from build123d import *

# Parameters (mm, degrees)
BOSS_EXTRUDE1_DEPTH = 5
SKETCH2_R           = 1.95
SKETCH2_W           = 40
SKETCH2_H           = 20
CUT_EXTRUDE1_DEPTH  = 6
SKETCH4_W           = 22
SKETCH4_H           = 49.22
CUT_EXTRUDE2_DEPTH  = 10
FILLET1_R           = 2
FILLET2_R           = 2
FILLET3_R           = 2
FILLET4_R           = 2
SKETCH5_R           = 1.95
SKETCH5_R_2         = 2
CUT_EXTRUDE3_DEPTH  = 6


with BuildPart() as part:
    # Sketch1 → Boss-Extrude1 (new body)
    with BuildSketch(Plane(origin=(0, 0, 0), x_dir=(1, 0, 0), z_dir=(0, 1, 0))):
        with BuildLine():
            Line((2, 0), (98, 0))
            ThreePointArc((98, 0), (99.414213562, -0.585786438), (100, -2))
            Line((100, -2), (100, -47.22))
            ThreePointArc((100, -47.22), (99.414213562, -48.634213562), (98, -49.22))
            Line((98, -49.22), (2, -49.22))
            ThreePointArc((2, -49.22), (0.585786438, -48.634213562), (0, -47.22))
            Line((0, -47.22), (0, -2))
            ThreePointArc((0, -2), (0.585786438, -0.585786438), (2, 0))
        make_face()
    extrude(amount=BOSS_EXTRUDE1_DEPTH)

    # Sketch2 → Cut-Extrude1 (cut, through all)
    with BuildSketch(Plane(origin=(0, 5, 0), x_dir=(1, 0, 0), z_dir=(0, 1, 0))):
        with Locations((90, -4.00475022)):
            Circle(SKETCH2_R)
        with Locations((82, -4.00475022)):
            Circle(SKETCH2_R)
        with Locations((18, -4.00475022)):
            Circle(SKETCH2_R)
        with Locations((26, -4.00475022)):
            Circle(SKETCH2_R)
        with Locations((34, -4.00475022)):
            Circle(SKETCH2_R)
        with Locations((42, -4.00475022)):
            Circle(SKETCH2_R)
        with Locations((50, -4.00475022)):
            Circle(SKETCH2_R)
        with Locations((58, -4.00475022)):
            Circle(SKETCH2_R)
        with Locations((66, -4.00475022)):
            Circle(SKETCH2_R)
        with Locations((74, -4.00475022)):
            Circle(SKETCH2_R)
        with Locations((90, -45.22)):
            Circle(SKETCH2_R)
        with Locations((82, -45.22)):
            Circle(SKETCH2_R)
        with Locations((18, -45.22)):
            Circle(SKETCH2_R)
        with Locations((26, -45.22)):
            Circle(SKETCH2_R)
        with Locations((34, -45.22)):
            Circle(SKETCH2_R)
        with Locations((42, -45.22)):
            Circle(SKETCH2_R)
        with Locations((50, -45.22)):
            Circle(SKETCH2_R)
        with Locations((58, -45.22)):
            Circle(SKETCH2_R)
        with Locations((66, -45.22)):
            Circle(SKETCH2_R)
        with Locations((74, -45.22)):
            Circle(SKETCH2_R)
        with Locations((50, -24.61)):
            Rectangle(SKETCH2_W, SKETCH2_H)
    extrude(amount=-CUT_EXTRUDE1_DEPTH, mode=Mode.SUBTRACT)

    # Sketch4 → Cut-Extrude2 (cut)
    with BuildSketch(Plane(origin=(0, 5, 0), x_dir=(1, 0, 0), z_dir=(0, 1, 0))):
        with Locations((89, -24.61)):
            Rectangle(SKETCH4_W, SKETCH4_H)
        with Locations((11, -24.61)):
            Rectangle(SKETCH4_W, SKETCH4_H)
    extrude(amount=-CUT_EXTRUDE2_DEPTH, mode=Mode.SUBTRACT)

    # Fillet1
    fillet1_edges = [part.edges().sort_by_distance(p)[0] for p in [
        (22, 2.5, 0),
    ]]
    fillet(fillet1_edges, radius=FILLET1_R)

    # Fillet2
    fillet2_edges = [part.edges().sort_by_distance(p)[0] for p in [
        (22, 2.5, 49.22),
    ]]
    fillet(fillet2_edges, radius=FILLET2_R)

    # Fillet3
    fillet3_edges = [part.edges().sort_by_distance(p)[0] for p in [
        (78, 2.5, 49.22),
    ]]
    fillet(fillet3_edges, radius=FILLET3_R)

    # Fillet4
    fillet4_edges = [part.edges().sort_by_distance(p)[0] for p in [
        (78, 2.5, 0),
    ]]
    fillet(fillet4_edges, radius=FILLET4_R)

    # Sketch5 → Cut-Extrude3 (cut, through all)
    with BuildSketch(Plane(origin=(0, 5, 0), x_dir=(1, 0, 0), z_dir=(0, 1, 0))):
        with Locations((74, -19.610250006)):
            Circle(SKETCH5_R)
        with Locations((73.9, -29.609749994)):
            Circle(SKETCH5_R_2)
        with Locations((26, -19.610250006)):
            Circle(SKETCH5_R)
        with Locations((26.1, -29.609749994)):
            Circle(SKETCH5_R_2)
    extrude(amount=-CUT_EXTRUDE3_DEPTH, mode=Mode.SUBTRACT)


solid = part.part
Read the model definition and answer for the solid it produces. Units are mm, in the model's axes. A direction names the side the tool comes from. Round coordinates to 2 decimals unless told otherwise and drop trailing zeros. Write each loop counter-clockwise with the first axis right and the second up, starting at its lowest first coordinate (ties: lowest second). Pieces come first, ordered by that corner, then holes. Notation, with made-up numbers: M -0.75,-1 L 8.25,-1 A24 cw 8.25,21 Z; hole C 27,35 d9. An arc over 180 degrees is marked long. Use a Markdown table: item, result.
1) For a pull along X with two mould halves and no side action, classify faces 3 (the cylindrical face through (22.57, 2.46, 48.62)), 4 (the flat face through (50, 2, 0)), 5 (the cylindrical face through (72.426, 2.535, 28.258)) as pulls with the +X half, pulls with the -X half, needs draft (parallel to the pull), parting line crosses it, or undercut.
Answers follow:
| item | result |
|---|---|
| face 3 | pulls with the -X half |
| face 4 | needs draft |
| face 5 | undercut |
2) The part is cut by section A-A (x = 42). Write down the section's boundary in (y, z), plus the area to 3 significant figures.
Answers follow:
| item | result |
|---|---|
| outline | M 0,0 L 5,0 L 5,2.05 L 0,2.05 Z; M 0,5.95 L 5,5.95 L 5,14.61 L 0,14.61 Z; M 0,34.61 L 5,34.61 L 5,43.27 L 0,43.27 Z; M 0,47.17 L 5,47.17 L 5,49.22 L 0,49.22 Z |
| area | 107 mm2 |
3) A tool of negligible diameter and unlimited length cuts with its end or side. For faces 1 (the flat face through (50, 3, 14.61)), 2 (the cylindrical face through (77.43, 2.46, 0.6)), from which of +Z, -Z, +X, -X, +Y, -Y can it reach the whole face along a straight path? Write none if from no direction.
Answers follow:
| item | result |
|---|---|
| face 1 | +Y, -Y |
| face 2 | -Z, +X, +Y, -Y |
4) Straight lines are drawn through the part: line 1 along Z through (x, y) = (34, 3.6); line 2 along Z through (x, y) = (26, 3.75); line 3 along X through (y, z) = (2.8, 34). For each, find the intervals that lie inside material, in ascending order. Write a range as [from, to].
Answers follow:
| item | result |
|---|---|
| line 1 | z = [0, 2.05], [5.95, 14.61], [34.61, 43.27], [47.17, 49.22] |
| line 2 | z = [0, 2.05], [5.95, 17.66], [21.56, 27.61], [31.61, 43.27], [47.17, 49.22] |
| line 3 | x = [22, 30], [70, 78] |
5) The part is cut by section B-B (z = 34). Write down the section's boundary in (x, y).
Answers follow:
| item | result |
|---|---|
| outline | M 22,0 L 30,0 L 30,5 L 22,5 Z; M 70,0 L 78,0 L 78,5 L 70,5 Z |
6) The part is cut by section C-C (x = 62.5). Write down the section's boundary in (y, z).
Answers follow:
| item | result |
|---|---|
| outline | M 0,0 L 5,0 L 5,14.61 L 0,14.61 Z; M 0,34.61 L 5,34.61 L 5,49.22 L 0,49.22 Z |
7) The part is cut by section D-D (y = 1.95). Give the number of separate pieces and of enclosed holes in the cut face, plus the area to 3 significant figures.
Answers follow:
| item | result |
|---|---|
| separate pieces | 1 |
| enclosed holes | 19 |
| area | 1,740 mm2 |
